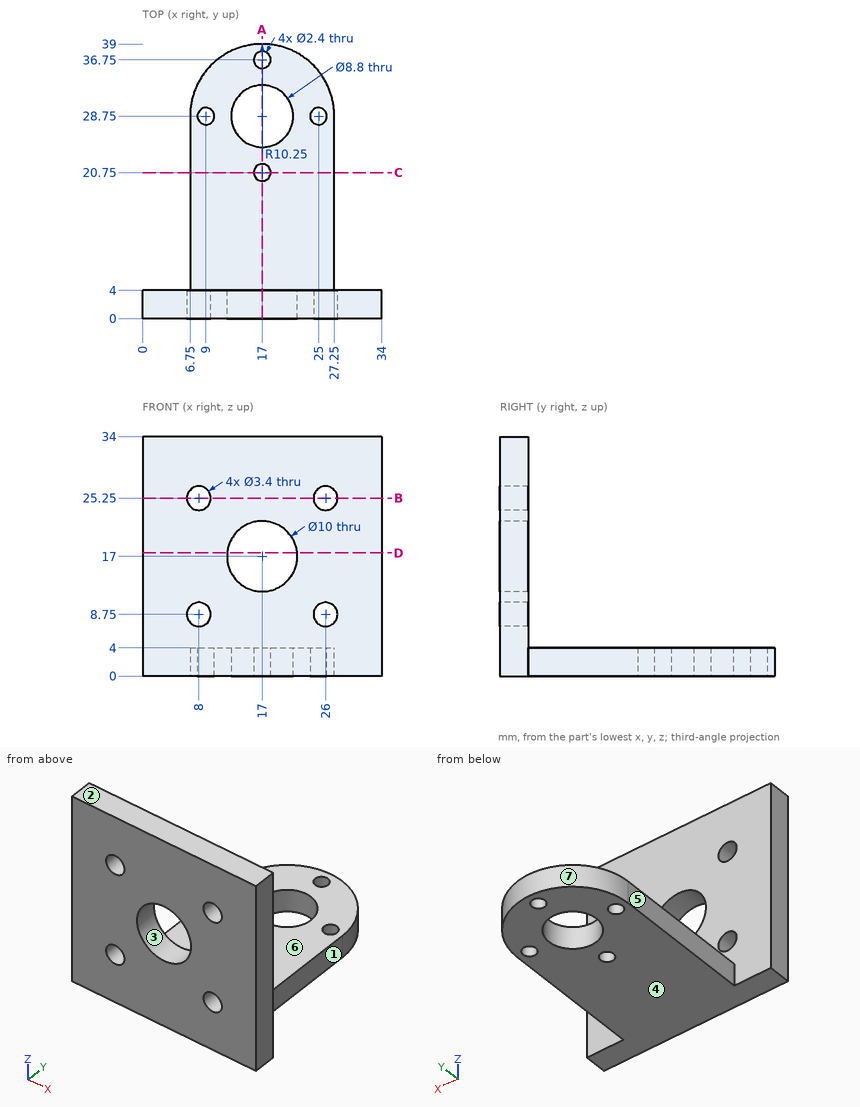
Geometry: see drawing. Coordinates: mm, zero at the bounding-box minimum. A direction names the side the tool comes from. Give positions to 0.01 mm unless a question says otherwise; leave off trailing zeros. Order: outer loops, then holes, each group sorted by start corner. A loop starts at its lowest first (then second) coordinate and runs counter-clockwise, first axis right, second up. Notation, with made-up numbers: (-37.75, 26.5) - (-22.75, 26.5) arc R17 cw to (-22.75, 42.5) - close; hole circle Ø2 at (10, 14.25). An arc over 180 degrees is marked (long way). Use a Markdown table: item, result.
(1) Line query: line 1 (Z direction, x = 8, y = 2); line 2 (Y direction, x = 17, z = 2.95); line 3 (Y direction, x = 4, z = 17). Output: solid intervals per line, ascending. Write a range as from..to.
Computed values:
| item | result |
|---|---|
| line 1 | z = 0..7.05, 10.45..23.55, 26.95..34 |
| line 2 | y = 0..19.55, 21.95..24.35, 33.15..35.55, 37.95..39 |
| line 3 | y = 0..4 |
(2) Section query D-D (z = 17.5). Output: boundary loops of the cut face in (x, y).
Computed values:
| item | result |
|---|---|
| outline | (0, 0) - (12.03, 0) - (12.03, 4) - (0, 4) - close; (21.97, 0) - (34, 0) - (34, 4) - (21.97, 4) - close |
(3) Section query A-A (x = 17). Output: boundary loops of the cut face in (y, z), then the cut area to 3 significant figures.
Computed values:
| item | result |
|---|---|
| outline | (0, 0) - (19.55, 0) - (19.55, 4) - (4, 4) - (4, 12) - (0, 12) - close; (0, 22) - (4, 22) - (4, 34) - (0, 34) - close; (21.95, 0) - (24.35, 0) - (24.35, 4) - (21.95, 4) - close; (33.15, 0) - (35.55, 0) - (35.55, 4) - (33.15, 4) - close; (37.95, 0) - (39, 0) - (39, 4) - (37.95, 4) - close |
| area | 182 mm2 |
(4) Pin query (flat end, axial travel): pin 1 (3 mm diameter, centred on x = 25, y = 28.75, fed in from -Z); pin 2 (3 mm diameter, centred on x = 12, z = 28, fed in from +Y); pin 3 (2 mm diameter, centred on y = 21.5, z = 1.5, fed in from +X); pin 4 (16.5 mm diameter, centred on x = 19.5, y = 23, fed in from +Z). Return the tip coordinate at first contact, or that it passes through.
Computed values:
| item | result |
|---|---|
| pin 1 | stops at z = 0 |
| pin 2 | stops at y = 4 |
| pin 3 | stops at x = 27.25 |
| pin 4 | stops at z = 4 |
(5) Section query B-B (z = 25.25). Output: boundary loops of the cut face in (x, y), then the cut area to 3 significant figures.
Computed values:
| item | result |
|---|---|
| outline | (0, 0) - (6.3, 0) - (6.3, 4) - (0, 4) - close; (9.7, 0) - (24.3, 0) - (24.3, 4) - (9.7, 4) - close; (27.7, 0) - (34, 0) - (34, 4) - (27.7, 4) - close |
| area | 109 mm2 |
(6) Draft query along Z for the marked faces 1, 2, 3 and 4. Return one class per face: released by +Z, released by -Z, zero draft, split by the parting line, or undercut.
Computed values:
| item | result |
|---|---|
| face 1 | zero draft |
| face 2 | released by +Z |
| face 3 | undercut |
| face 4 | released by -Z |
(7) Access query for the marked faces 5, 6 and 7. Directions: +Z, -Z, +X, -X, +Y, -Y. A direction counts if a zero-diameter tool reaches every point of the face in a straight line with its end or side. Return the directions, or none.
Computed values:
| item | result |
|---|---|
| face 5 | +Z, -Z, -X, +Y |
| face 6 | +Z, +X, -X, +Y |
| face 7 | +Z, -Z, +Y |
(8) Section query C-C (y = 20.75). Output: boundary loops of the cut face in (x, z), then the cut area to 3 significant figures.
Computed values:
| item | result |
|---|---|
| outline | (6.75, 0) - (15.8, 0) - (15.8, 4) - (6.75, 4) - close; (18.2, 0) - (27.25, 0) - (27.25, 4) - (18.2, 4) - close |
| area | 72.4 mm2 |
